```python
from build123d import *

# Parameters (mm, degrees)
SKETCH2_R           = 30
BOSS_EXTRUDE2_DEPTH = 20
SKETCH2_5_R         = 30
SKETCH2_5_R_2       = 20
BOSS_EXTRUDE3_DEPTH = 25


with BuildPart() as part:
    # Sketch2 → Boss-Extrude2 (new body)
    with BuildSketch(Plane.XY):
        with BuildLine():
            Line((147.355012786, 249.542955804), (147.355012786, 272.222447728))
            Line((147.355012786, 272.222447728), (187.355012786, 272.222447728))
            Line((187.355012786, 272.222447728), (187.355012786, 282.222447728))
            Line((187.355012786, 282.222447728), (237.355012786, 282.222447728))
            ThreePointArc((237.355012786, 282.222447728), (265.639284034, 270.506718976), (277.355012786, 242.222447728))
            Line((277.355012786, 242.222447728), (277.355012786, 196.222447728))
            Line((277.355012786, 196.222447728), (267.355012786, 196.222447728))
            ThreePointArc((267.355012786, 196.222447728), (213.355012786, 142.222447728), (267.355012786, 88.222447728))
            Line((267.355012786, 88.222447728), (277.355012786, 88.222447728))
            Line((277.355012786, 88.222447728), (277.355012786, 42.222447728))
            ThreePointArc((277.355012786, 42.222447728), (265.639284034, 13.938176481), (237.355012786, 2.222447728))
            Line((237.355012786, 2.222447728), (187.355012786, 2.222447728))
            Line((187.355012786, 2.222447728), (187.355012786, 12.222447728))
            Line((187.355012786, 12.222447728), (147.355012786, 12.222447728))
            Line((147.355012786, 12.222447728), (147.355012786, 34.901939653))
            ThreePointArc((147.355012786, 34.901939653), (137.355012786, 72.222447728), (127.355012786, 34.901939653))
            Line((127.355012786, 34.901939653), (127.355012786, 12.222447728))
            Line((127.355012786, 12.222447728), (87.355012786, 12.222447728))
            Line((87.355012786, 12.222447728), (87.355012786, 2.222447728))
            Line((87.355012786, 2.222447728), (37.355012786, 2.222447728))
            ThreePointArc((37.355012786, 2.222447728), (9.070741539, 13.938176481), (-2.644987214, 42.222447728))
            Line((-2.644987214, 42.222447728), (-2.644987214, 88.222447728))
            Line((-2.644987214, 88.222447728), (7.355012786, 88.222447728))
            ThreePointArc((7.355012786, 88.222447728), (61.355012786, 142.222447728), (7.355012786, 196.222447728))
            Line((7.355012786, 196.222447728), (-2.644987214, 196.222447728))
            Line((-2.644987214, 196.222447728), (-2.644987214, 242.222447728))
            ThreePointArc((-2.644987214, 242.222447728), (9.070741539, 270.506718976), (37.355012786, 282.222447728))
            Line((37.355012786, 282.222447728), (87.355012786, 282.222447728))
            Line((87.355012786, 282.222447728), (87.355012786, 272.222447728))
            Line((87.355012786, 272.222447728), (127.355012786, 272.222447728))
            Line((127.355012786, 272.222447728), (127.355012786, 249.542955804))
            ThreePointArc((127.355012786, 249.542955804), (137.355012786, 212.222447728), (147.355012786, 249.542955804))
        make_face()
        with Locations((237.355012786, 242.222447728)):
            Circle(SKETCH2_R, mode=Mode.SUBTRACT)
        with Locations((37.355012786, 42.222447728)):
            Circle(SKETCH2_R, mode=Mode.SUBTRACT)
        with Locations((37.355012786, 242.222447728)):
            Circle(SKETCH2_R, mode=Mode.SUBTRACT)
        with Locations((237.355012786, 42.222447728)):
            Circle(SKETCH2_R, mode=Mode.SUBTRACT)
    extrude(amount=BOSS_EXTRUDE2_DEPTH)

    # Sketch2_5 → Boss-Extrude3 (add)
    # profile 1 of 4: a face of its own
    with BuildSketch(Plane.XY):
        with Locations((37.355012786, 242.222447728)):
            Circle(SKETCH2_5_R)
        with Locations((37.355012786, 242.222447728)):
            Circle(SKETCH2_5_R_2, mode=Mode.SUBTRACT)
    # profile 2 of 4: a face of its own
    with BuildSketch(Plane.XY):
        with Locations((237.355012786, 242.222447728)):
            Circle(SKETCH2_5_R)
        with Locations((237.355012786, 242.222447728)):
            Circle(SKETCH2_5_R_2, mode=Mode.SUBTRACT)
    # profile 3 of 4: a face of its own
    with BuildSketch(Plane.XY):
        with Locations((37.355012786, 42.222447728)):
            Circle(SKETCH2_5_R)
        with Locations((37.355012786, 42.222447728)):
            Circle(SKETCH2_5_R_2, mode=Mode.SUBTRACT)
    # profile 4 of 4: a face of its own
    with BuildSketch(Plane.XY):
        with Locations((237.355012786, 42.222447728)):
            Circle(SKETCH2_5_R)
        with Locations((237.355012786, 42.222447728)):
            Circle(SKETCH2_5_R_2, mode=Mode.SUBTRACT)
    extrude(amount=BOSS_EXTRUDE3_DEPTH)


solid = part.part
```
The model under review builds one solid part; all positions refer to its coordinate system, in mm. A direction names the side the tool comes from. Round coordinates to 2 decimals unless told otherwise and drop trailing zeros. Order: outer loops, then holes, each group sorted by start corner. A loop starts at its lowest first (then second) coordinate and runs counter-clockwise, first axis right, second up. Notation, with made-up numbers: (34, 42.5) - (45, 42.5) arc R28 cw to (45, 75.5) - close; hole circle Ø11 at (82.25, 51). An arc over 180 degrees is marked (long way). Answer in a Markdown table with one row per item.
(1) Machinability: for faces 4 (the face through (2, 196.222, 10)), 5 (the face through (108, 12.222, 10)), 6 (the face through (107, 272.222, 10)), 7 (the face through (30.852, 212.936, 22.465)), 8 (the face through (272, 196.222, 10)), which of the approach directions +Z, -Z, +X, -X, +Y, -Y give a long, thin tool a straight path to every point of the face, cutting with its end or side? Answer none if there is none.
Result set:
| item | result |
|---|---|
| face 4 | +Z, -Z, -X |
| face 5 | +Z, -Z, -Y |
| face 6 | +Z, -Z, +Y |
| face 7 | +Z |
| face 8 | +Z, -Z, +X |
(2) Take a section at B-B on x = 52. Write out the cut boundary in (y, z).
Result set:
| item | result |
|---|---|
| outline | (2.22, 0) - (28.6, 0) - (28.6, 25) - (16.04, 25) - (16.04, 20) - (2.22, 20) - close; (55.84, 0) - (111.84, 0) - (111.84, 20) - (68.4, 20) - (68.4, 25) - (55.84, 25) - close; (172.6, 0) - (228.6, 0) - (228.6, 25) - (216.04, 25) - (216.04, 20) - (172.6, 20) - close; (255.84, 0) - (282.22, 0) - (282.22, 20) - (268.4, 20) - (268.4, 25) - (255.84, 25) - close |
(3) For line 1 (Y direction, x = 20, z = 13); line 2 (X direction, y = 230, z = 5); line 3 (Y direction, x = 53.5, z = 6.5), list the stretches that pass through material, from the lowest coordinate up. Write a range as from..to.
Result set:
| item | result |
|---|---|
| line 1 | y = 6.18..32.28, 52.16..89.72, 194.72..232.28, 252.16..278.26 |
| line 2 | x = -2.64..21.52, 53.19..117.48, 157.23..221.52, 253.19..277.36 |
| line 3 | y = 2.22..30.42, 54.03..114.18, 170.27..230.42, 254.03..282.22 |
(4) Mouldability with a two-part tool opening along X and no side actions: class faces 1 (the face through (139, 144, 0)), 2 (the face through (187.355, 277, 10)), 3 (the face through (-2.645, 219, 10)) as released by +X, released by -X, zero draft, split by the parting line, or undercut.
Result set:
| item | result |
|---|---|
| face 1 | zero draft |
| face 2 | undercut |
| face 3 | released by -X |
(5) Clearance check with flat-ended pins moving along their axes: P1, Ø8, axis at y = 6, z = 10.5, coming from the +X side; P2, Ø2, axis at x = 168, z = 20, coming from the +Y side; P3, Ø2, axis at y = 175, z = 3, coming from the +X side. State where each tip first meets the part, or that it passes through.
Result set:
| item | result |
|---|---|
| P1 | stops at x = 261.06 |
| P2 | stops at y = 272.22 |
| P3 | stops at x = 225.22 |
(6) Take a section at D-D on y = 170. Write out the cut boundary in (x, z).
Result set:
| item | result |
|---|---|
| outline | (53.66, 0) - (221.05, 0) - (221.05, 20) - (53.66, 20) - close |
(7) Take a section at A-A on y = 225.5. Write out the cut boundary in (x, z).
Result set:
| item | result |
|---|---|
| outline | (-2.64, 0) - (26.38, 0) - (26.38, 25) - (12.45, 25) - (12.45, 20) - (-2.64, 20) - close; (48.33, 0) - (118.52, 0) - (118.52, 20) - (62.26, 20) - (62.26, 25) - (48.33, 25) - close; (156.19, 0) - (226.38, 0) - (226.38, 25) - (212.45, 25) - (212.45, 20) - (156.19, 20) - close; (248.33, 0) - (277.36, 0) - (277.36, 20) - (262.26, 20) - (262.26, 25) - (248.33, 25) - close |
(8) Take a section at C-C on z = 15.75. Count the separate pieces of the cut face and the enclosed holes in it, plus the area to 3 significant figures.
Result set:
| item | result |
|---|---|
| separate pieces | 1 |
| enclosed holes | 4 |
| area | 55,300 mm2 |
